Can you work these out from the model? Positions are in its coordinate system, mm. A direction names the side the tool comes from. Coordinates: 2 decimals unless noted, no trailing zeros. Order: outer loops, then holes, each group sorted by start corner. A loop starts at its lowest first (then second) coordinate and runs counter-clockwise, first axis right, second up. Notation, with made-up numbers: (28, 33.5) -> (51, 33.5) arc R23 ccw to (51, 60.5) -> close; hole circle Ø1 at (-16.75, -4.75). An arc over 180 degrees is marked (long way). Use a Markdown table: item, result. Add a question column.
1. If I drill on line 1 along X through (y, z) = (-4.25, -68); line 2 along Z through (x, y) = (-140, -4); line 3 along Z through (x, y) = (-74, -4.75), over which ranges is the centre line in solid material (lowest first)? Write a range as from..to.
2. We'd pull the mould along Z, two halves only. Please class faces 3 (the flat face through (170, -4, 24)), 4 (the flat face through (-159.86, -4.437, -92.745)), 5 (the flat face through (-77, -4, -1)): pulls with the +Z half, pulls with the -Z half, needs draft (parallel to the pull), parting line crosses it, or undercut.
3. Suppose I cut it at B-B, the plane y = -2. State how many separate pieces and enclosed holes the cut face has, then the cut area to 3 significant figures.
4. Suppose I cut it at A-A, the plane x = -120. List the corners of the cut face in (y, z) for me, then the cut area to 3 significant figures.
5. For faces 1 (the flat face through (-107, -4, -50)), 2 (the flat face through (-170, -4, 21)), which set-ups out of +Z, -Z, +X, -X, +Y, -Y let a thin tool reach every point of the face, with its end or its side?
```python
from build123d import *

# Parameters (mm, degrees)
ESQUISSE3_R             = 2.55
STRUCTURE_DEPTH         = 9
ESQUISSE4_R             = 10
ESQUISSE4_R_2           = 11.5
ESQUISSE4_R_3           = 2.05
ESQUISSE4_R_4           = 6
ENL_V_MAT_EXTRU_1_DEPTH = 10
ESQUISSE5_OUTSIDE_W     = 424.118
ESQUISSE5_OUTSIDE_H     = 314.118
ESQUISSE5_OUTSIDE_R     = 2.55
ESQUISSE5_OUTSIDE_R_2   = 2.05
ENL_V_MAT_EXTRU_2_DEPTH = 10
ESQUISSE6_R             = 1.55
ENL_V_MAT_EXTRU_3_DEPTH = 209.281060109


with BuildPart() as part:
    # Esquisse3 → structure (new body)
    with BuildSketch(Plane(origin=(0, 0, 0), x_dir=(1, 0, 0), z_dir=(0, 1, 0))):
        Polygon((-170, 0), (-170, -120), (170, -120), (170, 0), (170, 75), (150, 110), (-150, 110), (-170, 75), align=None)
        with Locations(Location((-140, -80, 0), (0, 0, 270))):
            Circle(ESQUISSE3_R, mode=Mode.SUBTRACT)
        with Locations(Location((-140, 80, 0), (0, 0, 270))):
            Circle(ESQUISSE3_R, mode=Mode.SUBTRACT)
        with Locations(Location((140, -80, 0), (0, 0, 270))):
            Circle(ESQUISSE3_R, mode=Mode.SUBTRACT)
        with Locations(Location((140, 80, 0), (0, 0, 270))):
            Circle(ESQUISSE3_R, mode=Mode.SUBTRACT)
    extrude(amount=-STRUCTURE_DEPTH)

    # Esquisse4 → Enlèv. mat.-Extru.1 (cut)
    with BuildSketch(Plane(origin=(0, 0, 0), x_dir=(1, 0, 0), z_dir=(0, 1, 0))):
        with Locations(Location((0, 0, 0), (0, 0, 270))):
            Circle(ESQUISSE4_R)
        with Locations(Location((0, -90, 0), (0, 0, 270))):
            Circle(ESQUISSE4_R_2)
        with Locations(Location((0, 40, 0), (0, 0, 270))):
            Circle(ESQUISSE4_R_3)
        with Locations(Location((40, 0, 0), (0, 0, 270))):
            Circle(ESQUISSE4_R_3)
        with Locations(Location((0, -40, 0), (0, 0, 270))):
            Circle(ESQUISSE4_R_3)
        with Locations(Location((-40, 0, 0), (0, 0, 270))):
            Circle(ESQUISSE4_R_3)
        with Locations(Location((0, 80, 0), (0, 0, 270))):
            Circle(ESQUISSE4_R_4)
    extrude(amount=-ENL_V_MAT_EXTRU_1_DEPTH, mode=Mode.SUBTRACT)

    # Esquisse5 outside → Enlèv. mat.-Extru.2 (cut)
    # profile 1 of 9: a face of its own
    with BuildSketch(Plane(origin=(0, 0, 0), x_dir=(1, 0, 0), z_dir=(0, 1, 0))):
        with Locations((0, -5)):
            Rectangle(ESQUISSE5_OUTSIDE_W, ESQUISSE5_OUTSIDE_H)
        Polygon((-170, 75), (-170, -120), (170, -120), (170, 75), (150, 110), (-150, 110), align=None, mode=Mode.SUBTRACT)
    # profile 2 of 9: a face of its own
    with BuildSketch(Plane(origin=(0, 0, 0), x_dir=(1, 0, 0), z_dir=(0, 1, 0))):
        with Locations(Location((-140, 80, 0), (0, 0, 270))):
            Circle(ESQUISSE5_OUTSIDE_R)
    # profile 3 of 9: a face of its own
    with BuildSketch(Plane(origin=(0, 0, 0), x_dir=(1, 0, 0), z_dir=(0, 1, 0))):
        with Locations(Location((-140, -80, 0), (0, 0, 270))):
            Circle(ESQUISSE5_OUTSIDE_R)
    # profile 4 of 9: a face of its own
    with BuildSketch(Plane(origin=(0, 0, 0), x_dir=(1, 0, 0), z_dir=(0, 1, 0))):
        with Locations(Location((-136, 100, 0), (0, 0, 270))):
            Circle(ESQUISSE5_OUTSIDE_R_2)
    # profile 5 of 9: a face of its own
    with BuildSketch(Plane(origin=(0, 0, 0), x_dir=(1, 0, 0), z_dir=(0, 1, 0))):
        with Locations(Location((-160, 68, 0), (0, 0, 270))):
            Circle(ESQUISSE5_OUTSIDE_R_2)
    # profile 6 of 9: a face of its own
    with BuildSketch(Plane(origin=(0, 0, 0), x_dir=(1, 0, 0), z_dir=(0, 1, 0))):
        with Locations(Location((-160, -85, 0), (0, 0, 270))):
            Circle(ESQUISSE5_OUTSIDE_R_2)
    # profile 7 of 9: a face of its own
    with BuildSketch(Plane(origin=(0, 0, 0), x_dir=(1, 0, 0), z_dir=(0, 1, 0))):
        with Locations(Location((160, -85, 0), (0, 0, 270))):
            Circle(ESQUISSE5_OUTSIDE_R_2)
    # profile 8 of 9: a face of its own
    with BuildSketch(Plane(origin=(0, 0, 0), x_dir=(1, 0, 0), z_dir=(0, 1, 0))):
        with Locations(Location((160, 68, 0), (0, 0, 270))):
            Circle(ESQUISSE5_OUTSIDE_R_2)
    # profile 9 of 9: a face of its own
    with BuildSketch(Plane(origin=(0, 0, 0), x_dir=(1, 0, 0), z_dir=(0, 1, 0))):
        with Locations(Location((136, 100, 0), (0, 0, 270))):
            Circle(ESQUISSE5_OUTSIDE_R_2)
    extrude(amount=-ENL_V_MAT_EXTRU_2_DEPTH, mode=Mode.SUBTRACT)

    # Esquisse6 → Enlèv. mat.-Extru.3 (cut, through all)
    with BuildSketch(Plane(origin=(0, 0, 0), x_dir=(1, 0, 0), z_dir=(0, 1, 0))):
        with Locations(Location((-140, 45, 0), (0, 0, 270))):
            Circle(ESQUISSE6_R)
        with Locations(Location((-74, 45, 0), (0, 0, 270))):
            Circle(ESQUISSE6_R)
        with Locations(Location((-140, -45, 0), (0, 0, 270))):
            Circle(ESQUISSE6_R)
        with Locations(Location((-74, -45, 0), (0, 0, 270))):
            Circle(ESQUISSE6_R)
        with BuildLine():
            Line((-78, -50), (-136, -50))
            ThreePointArc((-136, -50), (-136.707106781, -49.707106781), (-137, -49))
            Line((-137, -49), (-137, 49))
            ThreePointArc((-137, 49), (-136.707106781, 49.707106781), (-136, 50))
            Line((-136, 50), (-78, 50))
            ThreePointArc((-78, 50), (-77.292893219, 49.707106781), (-77, 49))
            Line((-77, 49), (-77, -49))
            ThreePointArc((-77, -49), (-77.292893219, -49.707106781), (-78, -50))
        make_face()
    extrude(amount=-ENL_V_MAT_EXTRU_3_DEPTH, mode=Mode.SUBTRACT)


solid = part.part
```
Worked out:
| question | item | result |
|---|---|---|
| 1 | line 1 | x = -170..-162.05, -157.95..157.95, 162.05..170 |
| 1 | line 2 | z = -110..-82.55, -77.45..-46.55, -43.45..43.45, 46.55..77.45, 82.55..120 |
| 1 | line 3 | z = -110..-46.55, -43.45..43.45, 46.55..120 |
| 2 | face 3 | needs draft |
| 2 | face 4 | pulls with the -Z half |
| 2 | face 5 | undercut |
| 3 | separate pieces | 1 |
| 3 | enclosed holes | 22 |
| 3 | area | 70,400 mm² |
| 4 | outline | (-9, -110) -> (0, -110) -> (0, -50) -> (-9, -50) -> close; (-9, 50) -> (0, 50) -> (0, 120) -> (-9, 120) -> close |
| 4 | area | 1,170 mm² |
| 5 | face 1 | +Y, -Y |
| 5 | face 2 | +Z, -Z, -X, +Y, -Y |
